Geometry: final body of the model. Coordinates: model frame, mm. Face numbers are marked on the shaded views. Give positions to 0.01 mm unless a question says otherwise; leave off trailing zeros. Loops run counter-clockwise (first coordinate to the right, second up) from the corner with the lowest first, then second, coordinate; pieces in that order, holes last. Notation, with made-up numbers: (69, 56) -> (127, 56) arc R28 cw to (127, 76) -> close; hole circle Ø4 at (-11.75, 44). An arc over 180 degrees is marked (long way). One line per question, with ' | ' between items. Start each with the question number.
Item 1: Section D-D on x = 67.5. Return loops of the section in (y, z).
Item 2: Mould query, pull axis Y, two halves, no side actions, for the marked faces 1, 2 and 3. Classes: released by +Y, released by -Y, zero draft, split by the parting line, or undercut.
Item 3: Section A-A on x = -10. Return loops of the section in (y, z), then the cut area to 3 significant figures.
Item 4: Pin query (flat end, axial travel): P1, Ø1, axis at x = 42.5, z = 3, coming from the +Y side; P2, Ø1, axis at y = 67, z = 10, coming from the -X side; P3, Ø8, axis at x = 19, z = 10.5, coming from the +Y side. Return the tip coordinate at first contact, or that it passes through.
Item 5: Material intervals for line 1 along Y through (x, z) = (-0.5, 2.5); line 2 along X through (y, z) = (39, 12.25); line 3 along X through (y, z) = (24, 2), sorted ascending. Write a range as [from, to].
Item 6: Section C-C on y = 31. Return loops of the section in (x, z), then the cut area to 3 significant figures.
Item 7: Section B-B on z = 12.25. Return loops of the section in (x, y), then the cut area to 3 significant figures.
from build123d import *

# Parameters (mm, degrees)
SKETCH1_R           = 17.5
SKETCH1_R_2         = 3.25
BOSS_EXTRUDE1_DEPTH = 15


with BuildPart() as part:
    # Sketch1 → Boss-Extrude1 (new body)
    with BuildSketch(Plane.XY):
        with BuildLine():
            Line((149.99990581, 70.000115429), (79.694106831, 87.00526078))
            Line((79.694106831, 87.00526078), (-1.24795586, 84.984541416))
            ThreePointArc((-1.24795586, 84.984541416), (-45.852560512, 15.061426098), (35.707047952, 0.000115429))
            Line((35.707047952, 0.000115429), (149.99990581, 0.000115429))
            Line((149.99990581, 0.000115429), (149.99990581, 70.000115429))
        make_face()
        with Locations((-9.419e-05, 35.000115429)):
            Circle(SKETCH1_R, mode=Mode.SUBTRACT)
        with Locations((79.694106831, 77.479356086)):
            Circle(SKETCH1_R_2, mode=Mode.SUBTRACT)
    extrude(amount=BOSS_EXTRUDE1_DEPTH)


solid = part.part
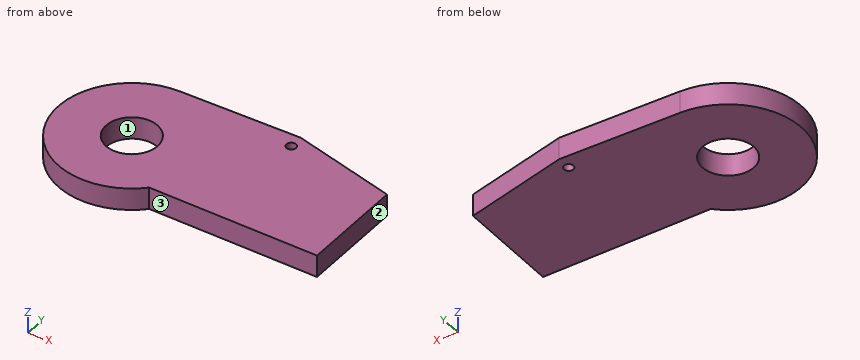
Result sheet:
1) outline: (0, 0) -> (86.7, 0) -> (86.7, 15) -> (0, 15) -> close
2) face 1: undercut | face 2: zero draft | face 3: released by -Y
3) outline: (-13.99, 0) -> (20.64, 0) -> (20.64, 15) -> (-13.99, 15) -> close; (49.36, 0) -> (83.99, 0) -> (83.99, 15) -> (49.36, 15) -> close | area: 1,040 mm²
4) P1: stops at y = 86.09 | P2: stops at x = -38.83 | P3: stops at y = 85.59
5) line 1: y = [-15, 17.51], [52.49, 85] | line 2: x = [-49.84, -17.04], [17.04, 150] | line 3: x = [-48.78, -13.61], [13.61, 150]
6) outline: (-49.84, 0) -> (-17.04, 0) -> (-17.04, 15) -> (-49.84, 15) -> close; (17.04, 0) -> (150, 0) -> (150, 15) -> (17.04, 15) -> close | area: 2,490 mm²
7) outline: (-1.25, 84.98) arc R50 ccw (long way) to (35.71, 0) -> (150, 0) -> (150, 70) -> (79.69, 87.01) -> close; hole circle Ø35 at (0, 35); hole circle Ø6.5 at (79.69, 77.48) | area: 15,700 mm²
